Read the model definition and answer for the solid it produces. Units are mm, in the model's axes. A direction names the side the tool comes from. Give positions to 0.01 mm unless a question says otherwise; leave off trailing zeros. Order: outer loops, then holes, each group sorted by start corner. A loop starts at its lowest first (then second) coordinate and runs counter-clockwise, first axis right, second up. Notation, with made-up numbers: (36.25, -7.75) - (48.25, -7.75) arc R13 cw to (48.25, 10.25) - close; hole circle Ø5 at (28, 36). An arc over 180 degrees is marked (long way). Use a Markdown table: item, result. Add a question column.
1. Flat-ended cylindrical pins translate along their axes: P1, Ø3.5, axis at y = 1, z = -28.5, coming from the +X side; P2, Ø2.5, axis at x = 0.5, y = -1, coming from the +Z side; P3, Ø1.3, axis at y = -2, z = -30.5, coming from the -X side. Find the tip coordinate at first contact, or state that the pin passes through.
2. A cutting plane is placed at A-A on z = -10. Determine the outline of the cut face in (x, y).
3. A cutting plane is placed at C-C on y = 0. Determine the outline of the cut face in (x, z).
4. Consider L1, parallel to Y at x = 0.25, z = -10.5; L2, parallel to X at y = 2, z = -14.5; L3, parallel to Y at x = -3, z = -29. Determine where each line is inside the solid, lowest interval first.
5. A cutting plane is placed at B-B on x = -0.5. Determine the outline of the cut face in (y, z).
6. Which of the six approach directions +Z, -Z, +X, -X, +Y, -Y give full straight-line access (tool end or side, diameter ignored) to faces 5 (the flat face through (0, -4, -30)), 6 (the flat face through (6.5, 0, -7)), 7 (the flat face through (0, 4, -30))?
7. A cutting plane is placed at D-D on z = -30. Determine the outline of the cut face in (x, y), and give its area (3 significant figures).
8. For a pull along X with two mould halves and no side action, classify faces 1 (the flat face through (0, -3, 0)), 2 (the flat face through (-6.09, 0.07, -23.82)), 3 (the flat face through (0, -2.5, -7)), 4 (the flat face through (-6, -1, -9)) as released by +X, released by -X, zero draft, split by the parting line, or undercut.
```python
from build123d import *

# Parameters (mm, degrees)
EXTRUDE_1_DEPTH      = 8.5
EXTRUDE_1_DEPTH_BACK = 8.5
CUT_EXTRUDE_3_DEPTH  = 36.049964337
FILLET_3_R           = 0.5
SKETCH_3_W           = 13
SKETCH_3_H           = 5
CUT_EXTRUDE_1_DEPTH  = 15
SKETCH_4_W           = 12
SKETCH_4_H           = 1.5
EXTRUDE_2_DEPTH      = 13
FILLET_2_R           = 0.2


with BuildPart() as part:
    # 草图2 → 凸台-拉伸1 (new, two sides: drawn at the far end of the back side and taken through both)
    with BuildSketch(Plane(origin=(0, 0, 0), x_dir=(0, 0, -1), z_dir=(1, 0, 0)).offset(-EXTRUDE_1_DEPTH_BACK)):
        Polygon((0, -5), (0, 5), (20, 5), (27.532919446, 4), (32.5, 4), (32.5, -4), (27.532919446, -4), (20, -5), align=None)
    extrude(amount=EXTRUDE_1_DEPTH + EXTRUDE_1_DEPTH_BACK)

    # 草图5 → 切除-拉伸3 (cut, through all)
    with BuildSketch(Plane(origin=(0, 5, 0), x_dir=(1, 0, 0), z_dir=(0, 1, 0))):
        Polygon((-3.75, 32.5), (-3.75, 27.532919446), (-8.5, 20), (-8.5, 32.5), align=None)
        Polygon((8.5, 32.5), (3.75, 32.5), (3.75, 27.532919446), (8.5, 20), align=None)
    extrude(amount=-CUT_EXTRUDE_3_DEPTH, mode=Mode.SUBTRACT)

    # 圆角3
    fillet_3_edges = [part.edges().sort_by_distance(p)[0] for p in [
        (0, -5, 0),
        (0, 5, 0),
        (8.5, 0, 0),
        (0, -4, -32.5),
        (0, 4, -32.5),
        (-3.75, 0, -32.5),
        (-8.5, 0, 0),
        (3.75, 0, -32.5),
    ]]
    fillet(fillet_3_edges, radius=FILLET_3_R)

    # 草图3 → 切除-拉伸1 (cut)
    with BuildSketch(Plane.XY):
        Rectangle(SKETCH_3_W, SKETCH_3_H)
    extrude(amount=-CUT_EXTRUDE_1_DEPTH, mode=Mode.SUBTRACT)

    # 草图4 → 凸台-拉伸2 (add)
    with BuildSketch(Plane.XY.offset(-15)):
        with Locations((0, -1.25)):
            Rectangle(SKETCH_4_W, SKETCH_4_H)
    extrude(amount=EXTRUDE_2_DEPTH)

    # 圆角2
    fillet_2_edges = [part.edges().sort_by_distance(p)[0] for p in [
        (0, -0.5, -2),
        (-6, -1.25, -2),
        (0, -2, -2),
        (6, -1.25, -2),
    ]]
    fillet(fillet_2_edges, radius=FILLET_2_R)


solid = part.part
```
Output values:
| question | item | result |
|---|---|---|
| 1 | P1 | x = 4.24 |
| 1 | P2 | z = -2 |
| 1 | P3 | x = -3.75 |
| 2 | outline | (-8.5, -5) - (8.5, -5) - (8.5, 5) - (-8.5, 5) - close; (-6, -2) - (6, -2) - (6, -0.5) - (-6, -0.5) - close; hole (-6.5, -2.5) - (6.5, -2.5) - (6.5, 2.5) - (-6.5, 2.5) - close |
| 3 | outline | (-8.5, -20) - (-3.75, -27.53) - (-3.75, -32) arc R0.5 ccw to (-3.25, -32.5) - (3.25, -32.5) arc R0.5 ccw to (3.75, -32) - (3.75, -27.53) - (8.5, -20) - (8.5, -0.5) arc R0.5 ccw to (8, 0) - (6.5, 0) - (6.5, -15) - (-6.5, -15) - (-6.5, 0) - (-8, 0) arc R0.5 ccw to (-8.5, -0.5) - close |
| 4 | L1 | -5 to -2.5, -2 to -0.5, 2.5 to 5 |
| 4 | L2 | -8.5 to -6.5, 6.5 to 8.5 |
| 4 | L3 | -4 to 4 |
| 5 | outline | (-5, -20) - (-4, -27.53) - (-4, -32) arc R0.5 ccw to (-3.5, -32.5) - (3.5, -32.5) arc R0.5 ccw to (4, -32) - (4, -27.53) - (5, -20) - (5, -0.5) arc R0.5 ccw to (4.5, 0) - (2.5, 0) - (2.5, -15) - (-0.5, -15) - (-0.5, -2.2) arc R0.2 ccw to (-0.7, -2) - (-1.8, -2) arc R0.2 ccw to (-2, -2.2) - (-2, -15) - (-2.5, -15) - (-2.5, 0) - (-4.5, 0) arc R0.5 ccw to (-5, -0.5) - close |
| 6 | face 5 | -Z, +X, -X, -Y |
| 6 | face 6 | +Z |
| 6 | face 7 | -Z, +X, -X, +Y |
| 7 | outline | (-3.75, -4) - (3.75, -4) - (3.75, 4) - (-3.75, 4) - close |
| 7 | area | 60.0 mm² |
| 8 | face 1 | zero draft |
| 8 | face 2 | released by -X |
| 8 | face 3 | undercut |
| 8 | face 4 | undercut |
